Work out the finished part from the listing and answer in its coordinate system (mm). A direction names the side the tool comes from. Give positions to 0.01 mm unless a question says otherwise; leave off trailing zeros. Order: outer loops, then holes, each group sorted by start corner. A loop starts at its lowest first (then second) coordinate and runs counter-clockwise, first axis right, second up.
```python
from build123d import *

# Parameters (mm, degrees)
BOSS_EXTRUDE1_DEPTH = 115.316
SKETCH2_R           = 1.1938
CUT_EXTRUDE1_DEPTH  = 6.985
SKETCH2_4_R         = 1.1938
CUT_EXTRUDE2_DEPTH  = 6.985
SKETCH2_5_W         = 5.8674
SKETCH2_5_H         = 2.3876
CUT_EXTRUDE3_DEPTH  = 6.985
FILLET1_R           = 1.27
BOSS_EXTRUDE2_DEPTH = 0.0254
CUT_EXTRUDE5_DEPTH  = 0.0254


with BuildPart() as part:
    # Sketch1 → Boss-Extrude1 (new body)
    with BuildSketch(Plane.XY):
        Polygon((-15.875, -5.588), (15.875, -5.588), (19.6215, 0), (15.875, 5.588), (-15.875, 5.588), (-19.6215, 0), align=None)
    extrude(amount=BOSS_EXTRUDE1_DEPTH)

    # Sketch2 → Cut-Extrude1 (cut)
    with BuildSketch(Plane(origin=(0, 0, 0), x_dir=(-1, 0, 0), z_dir=(0, 0, -1))):
        with Locations((-2.9337, 0)):
            Circle(SKETCH2_R)
    extrude(amount=-CUT_EXTRUDE1_DEPTH, mode=Mode.SUBTRACT)

    # Sketch2_4 → Cut-Extrude2 (cut)
    with BuildSketch(Plane(origin=(0, 0, 0), x_dir=(-1, 0, 0), z_dir=(0, 0, -1))):
        with Locations(Location((2.9337, 0, 0), (0, 0, 180))):
            Circle(SKETCH2_4_R)
    extrude(amount=-CUT_EXTRUDE2_DEPTH, mode=Mode.SUBTRACT)

    # Sketch2_5 → Cut-Extrude3 (cut)
    with BuildSketch(Plane(origin=(0, 0, 0), x_dir=(-1, 0, 0), z_dir=(0, 0, -1))):
        Rectangle(SKETCH2_5_W, SKETCH2_5_H)
    extrude(amount=-CUT_EXTRUDE3_DEPTH, mode=Mode.SUBTRACT)

    # Fillet1
    fillet1_edges = [part.edges().sort_by_distance(p)[0] for p in [
        (-15.875, 5.588, 57.658),
        (15.875, 5.588, 57.658),
        (19.6215, 0, 57.658),
        (15.875, -5.588, 57.658),
        (-15.875, -5.588, 57.658),
        (-19.6215, 0, 57.658),
    ]]
    fillet(fillet1_edges, radius=FILLET1_R)

    # Sketch4 → Boss-Extrude2 (add)
    with BuildSketch(Plane(origin=(0, 5.588, 0), x_dir=(1, 0, 0), z_dir=(0, 1, 0))):
        Polygon((15.19745355, 0), (-15.19745355, 0), (-15.19745355, -5.715), (0, -19.558), (15.19745355, -5.715), align=None)
    boss_extrude2 = extrude(amount=BOSS_EXTRUDE2_DEPTH)

    # Mirror1: Boss-Extrude2 across plane
    add(boss_extrude2.mirror(Plane.ZX))

    # Sketch6 → Cut-Extrude5 (cut)
    with BuildSketch(Plane(origin=(0, 5.6134, 0), x_dir=(1, 0, 0), z_dir=(0, 1, 0))):
        Polygon((0, -17.018), (-6.009529828, -11.544061808), (0, -14.478), (6.009529828, -11.544061808), align=None)
    extrude(amount=-CUT_EXTRUDE5_DEPTH, mode=Mode.SUBTRACT)


solid = part.part
```
1. Which of the six approach directions +Z, -Z, +X, -X, +Y, -Y give full straight-line access (tool end or side, diameter ignored) to faces 1 (the face through (0, 1.194, 3)), 2 (the face through (0, 3, 0))?
Findings below:
face 1: -Z
face 2: -Z, +X, -X, +Y, -Y
2. Straight lines are drawn through the part: probe 1 along Y at (x, z) = (-12, 45.5); probe 2 along X at (y, z) = (0.5, 5); probe 3 along Z at (x, y) = (2, -1) (3 decimals). For each, find the intervals that lie inside material, in ascending order.
Findings below:
probe 1: y = -5.59 to 5.59
probe 2: x = -19.26 to -4.02, 4.02 to 19.26
probe 3: z = 6.985 to 115.316
3. Given P1, Ø5, axis at x = 9, z = 77.5, coming from the -Y side; P2, Ø15, axis at x = -7, z = 47.5, coming from the +Y side; P3, Ø3, axis at y = -3, z = 42.5, coming from the +X side, each flat-ended and moving along its own axis, determine where each tip first touches the part or whether it passes through.
Findings below:
P1: stops at y = -5.59
P2: stops at y = 5.59
P3: stops at x = 18.62
4. The part is cut by section B-B (y = 3). Write down the section's boundary in (x, z).
Findings below:
outline: (-17.61, 0) - (17.61, 0) - (17.61, 115.32) - (-17.61, 115.32) - close
5. The part is cut by section A-A (z = 63.5). Write down the section's boundary in (x, y), then the cut area to 3 significant figures.
Findings below:
outline: (-19.15, -0.71) - (-16.25, -5.03) arc R1.27 ccw to (-15.2, -5.59) - (15.2, -5.59) arc R1.27 ccw to (16.25, -5.03) - (19.15, -0.71) arc R1.27 ccw to (19.15, 0.71) - (16.25, 5.03) arc R1.27 ccw to (15.2, 5.59) - (-15.2, 5.59) arc R1.27 ccw to (-16.25, 5.03) - (-19.15, 0.71) arc R1.27 ccw to start
area: 396 mm2
